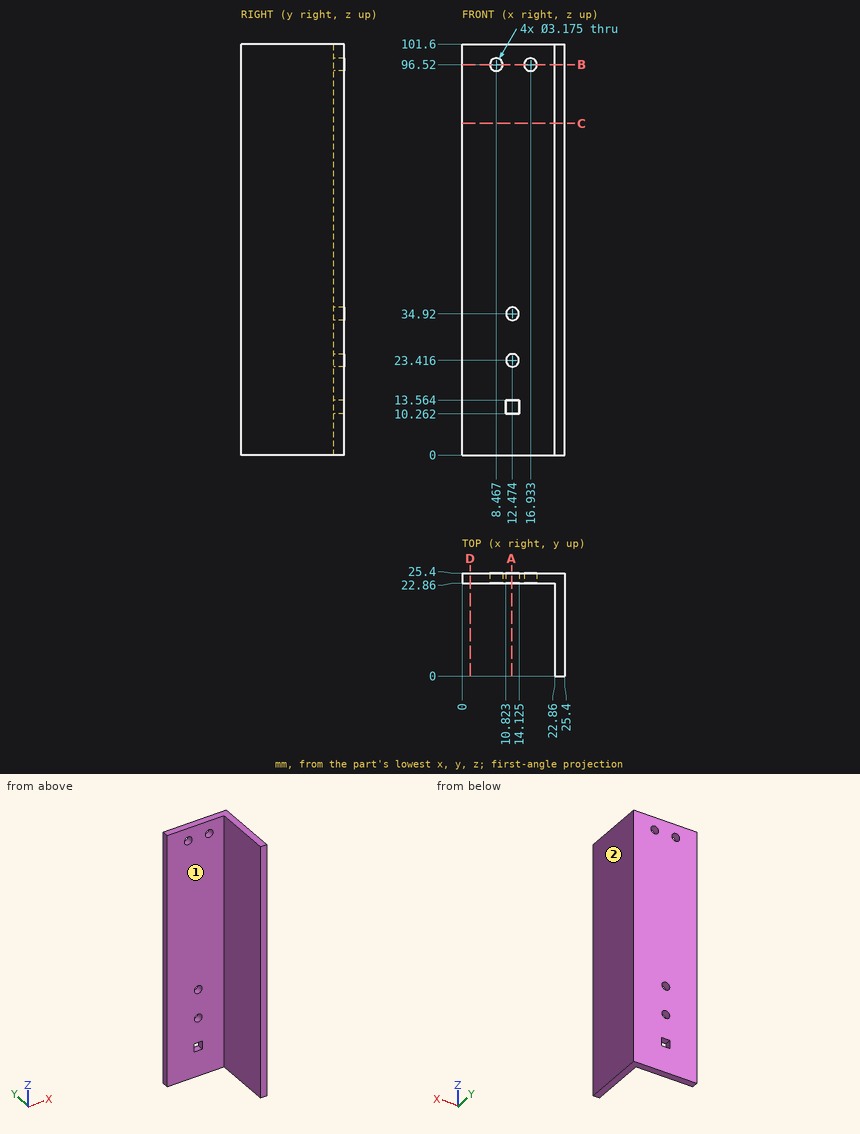
Geometry check sheet. Reference: drawing and pictorial views, mm from the part's lowest x, y, z. A direction names the side the tool comes from. Give positions to 0.01 mm unless a question says otherwise; leave off trailing zeros. Order: outer loops, then holes, each group sorted by start corner. A loop starts at its lowest first (then second) coordinate and runs counter-clockwise, first axis right, second up. Notation, with made-up numbers: M 64,49.5 L 106,49.5 A27 cw 106,77.5 Z; hole C -5,78 d1. An arc over 180 degrees is marked long. Answer as CSV lines item,"result". Start each with the question number.
Item 1: Cross-section at B-B on z = 96.52. Enter the section's corners in (x, y).
Item 2: Cross-section at D-D on x = 2. Enter the section's corners in (y, z), plus the area to 3 significant figures.
Item 3: Thickness scan on line 1 (X direction, y = 24.55, z = 96.52) (1 decimal); line 2 (X direction, y = 18.75, z = 88). Record the ranges inside material, lowest first. Write a range as [from, to].
Item 4: Cross-section at A-A on x = 12.25. Enter the section's corners in (y, z) (1 decimal).
Item 5: Tool access check on the marked faces 1 and 2. Record the directions out of +Z, -Z, +X, -X, +Y, -Y that give a thin tool (end or side, any length) a straight path to the whole face; none if there is none.
Item 6: Cross-section at C-C on z = 82. Enter the section's corners in (x, y).
Item 7: Gauge pin test, flat ends, axial feed: P1, Ø1, axis at x = 21, z = 17.5, coming from the -Y side; P2, Ø8, axis at y = 9, z = 76, coming from the -X side. Record the tip position at first contact, or that the pin passes through.
Established:
1,outline,"M 0,22.86 L 6.88,22.86 L 6.88,25.4 L 0,25.4 Z; M 10.05,22.86 L 15.35,22.86 L 15.35,25.4 L 10.05,25.4 Z; M 18.52,22.86 L 22.86,22.86 L 22.86,0 L 25.4,0 L 25.4,25.4 L 18.52,25.4 Z"
2,outline,"M 22.86,0 L 25.4,0 L 25.4,101.6 L 22.86,101.6 Z"
2,area,"258 mm^2"
3,line 1,"x = [0, 6.9], [10.1, 15.3], [18.5, 25.4]"
3,line 2,"x = [22.86, 25.4]"
4,outline,"M 22.9,0 L 25.4,0 L 25.4,10.3 L 22.9,10.3 Z; M 22.9,13.6 L 25.4,13.6 L 25.4,21.8 L 22.9,21.8 Z; M 22.9,25 L 25.4,25 L 25.4,33.3 L 22.9,33.3 Z; M 22.9,36.5 L 25.4,36.5 L 25.4,101.6 L 22.9,101.6 Z"
5,face 1,"+Z, -Z, -X, -Y"
5,face 2,"+Z, -Z, +X, +Y, -Y"
6,outline,"M 0,22.86 L 22.86,22.86 L 22.86,0 L 25.4,0 L 25.4,25.4 L 0,25.4 Z"
7,P1,"stops at y = 22.86"
7,P2,"stops at x = 22.86"
